```python
from build123d import *

# Parameters (mm, degrees)
SKETCH1_R           = 18.5
BOSS_EXTRUDE1_DEPTH = 26.5
SKETCH2_R           = 13.7
BOSS_EXTRUDE2_DEPTH = 38
SKETCH3_R           = 6
BOSS_EXTRUDE3_DEPTH = 6.8
SKETCH4_R           = 3
BOSS_EXTRUDE4_DEPTH = 30
SKETCH5_R           = 1.5
CUT_EXTRUDE1_DEPTH  = 6
CIRPATTERN1_COUNT   = 6
SKETCH6_R           = 13.75
BOSS_EXTRUDE5_DEPTH = 15
SKETCH7_R           = 1.5
CUT_EXTRUDE2_DEPTH  = 69.49372234


with BuildPart() as part:
    # Sketch1 → Boss-Extrude1 (new body)
    with BuildSketch(Plane.XY):
        Circle(SKETCH1_R)
    extrude(amount=BOSS_EXTRUDE1_DEPTH)

    # Sketch2 → Boss-Extrude2 (add)
    with BuildSketch(Plane(origin=(0, 0, 0), x_dir=(-1, 0, 0), z_dir=(0, 0, -1))):
        with Locations(Location((0, 0, 0), (0, 0, 180))):
            Circle(SKETCH2_R)
    extrude(amount=BOSS_EXTRUDE2_DEPTH)

    # Sketch3 → Boss-Extrude3 (add)
    with BuildSketch(Plane.XY.offset(26.5)):
        with Locations((0, 7)):
            Circle(SKETCH3_R)
    extrude(amount=BOSS_EXTRUDE3_DEPTH)

    # Sketch4 → Boss-Extrude4 (add)
    with BuildSketch(Plane.XY.offset(33.3)):
        with Locations((0, 7)):
            Circle(SKETCH4_R)
    extrude(amount=BOSS_EXTRUDE4_DEPTH)

    # Sketch5 → Cut-Extrude1 (cut)
    with BuildSketch(Plane.XY.offset(26.5)):
        with Locations((15.75, 0)):
            Circle(SKETCH5_R)
    cut_extrude1 = extrude(amount=-CUT_EXTRUDE1_DEPTH, mode=Mode.SUBTRACT)

    # CirPattern1: Cut-Extrude1 ×6 about axis
    cirpattern1_axis = Axis((0, 0, 0), (0, 0, 1))
    for i in range(1, CIRPATTERN1_COUNT):
        add(cut_extrude1.rotate(cirpattern1_axis, i * 360 / CIRPATTERN1_COUNT), mode=Mode.SUBTRACT)

    # Sketch6 → Boss-Extrude5 (add)
    with BuildSketch(Plane(origin=(0, 0, -38), x_dir=(-1, 0, 0), z_dir=(0, 0, -1))):
        Circle(SKETCH6_R)
    extrude(amount=BOSS_EXTRUDE5_DEPTH)

    # Sketch7 → Cut-Extrude2 (cut, through all)
    with BuildSketch(Plane(origin=(0, 0, 0), x_dir=(1, 0, 0), z_dir=(0, 1, 0))):
        with Locations(Location((0, -53.3, 0), (0, 0, 90))):
            Circle(SKETCH7_R)
    extrude(amount=CUT_EXTRUDE2_DEPTH, mode=Mode.SUBTRACT)


solid = part.part
```
The model under review builds one solid part; all positions refer to its coordinate system, in mm. A direction names the side the tool comes from. Round coordinates to 2 decimals unless told otherwise and drop trailing zeros. Write each loop counter-clockwise with the first axis right and the second up, starting at its lowest first coordinate (ties: lowest second). Pieces come first, ordered by that corner, then holes. Notation, with made-up numbers: (47.5, 34) - (74.5, 34) arc R3 ccw to (74.5, 39) - close; hole circle Ø1 at (26.5, -37). An arc over 180 degrees is marked (long way). Use one line per item in the form item = value.
Q1. For line 1 (Z direction, x = -6.5, y = 6.5); line 2 (Z direction, x = 4.5, y = 14); line 3 (X direction, y = 8.5, z = 53.3), list the stretches that pass through material, from the lowest coordinate up. Write a range as [from, to].
Answer key:
line_1 = [-53, 26.5]
line_2 = [0, 26.5]
line_3 = [-2.6, -1.5], [1.5, 2.6]
Q2. Consider section A-A (x = 0). State the section outline as (y, z) points, and give its area (3 significant figures).
Answer key:
outline = (-18.5, 0) - (-13.7, 0) - (-13.7, -38) - (-13.75, -38) - (-13.75, -53) - (13.75, -53) - (13.75, -38) - (13.7, -38) - (13.7, 0) - (18.5, 0) - (18.5, 26.5) - (13, 26.5) - (13, 33.3) - (10, 33.3) - (10, 51.8) - (4, 51.8) - (4, 33.3) - (1, 33.3) - (1, 26.5) - (-18.5, 26.5) - close; (4, 54.8) - (10, 54.8) - (10, 63.3) - (4, 63.3) - close
area = 2,680 mm2
Q3. Consider section B-B (y = 7). State the section outline as (x, z) points, and give its area (3 significant figures).
Answer key:
outline = (-17.12, 0) - (-11.78, 0) - (-11.78, -38) - (-11.83, -38) - (-11.83, -53) - (11.83, -53) - (11.83, -38) - (11.78, -38) - (11.78, 0) - (17.12, 0) - (17.12, 26.5) - (6, 26.5) - (6, 33.3) - (3, 33.3) - (3, 63.3) - (-3, 63.3) - (-3, 33.3) - (-6, 33.3) - (-6, 26.5) - (-17.12, 26.5) - close; hole circle Ø3 at (0, 53.3)
area = 2,410 mm2
Q4. Draft analysis for pull direction Z (two halves, no side actions). For faces 1 (the cylindrical face through (-1.265, 6.958, 52.494)), 2 (the flat face through (8, 14, 20.5)), state which applies: +Z half, -Z half, draft (parallel to the pull), parting line (faces both ways), or undercut.
Answer key:
face_1 = undercut
face_2 = +Z half
Q5. Consider section C-C (x = -10.5). State the section outline as (y, z) points.
Answer key:
outline = (-15.23, 0) - (-8.8, 0) - (-8.8, -38) - (-8.88, -38) - (-8.88, -53) - (8.88, -53) - (8.88, -38) - (8.8, -38) - (8.8, 0) - (15.23, 0) - (15.23, 26.5) - (-15.23, 26.5) - close
Q6. Tool access review of faces 3 (the cylindrical face through (-3, 7, 48)), 4 (the cylindrical face through (-4.01, -18.06, 13.06)): name each direction out of +Z, -Z, +X, -X, +Y, -Y from which nothing blocks a thin tool from reaching the whole face with its end or side.
Answer key:
face_3 = +Z
face_4 = +Z, -Z
Q7. Insertion check: pin 1 Ø2.5 at (x, y) = (-7.88, -13.64) entering from -Z; pin 2 Ø2.5 at (x, z) = (0, 53.3) entering from +Y; pin 3 Ø5 at (x, y) = (-15.75, 0) entering from +Z; pin 4 Ø10 at (x, z) = (8.5, -24) entering from +Y. Each pin has a flat end and moves straight along its axis. Give the tip position at first contact, or say it passes through.
Answer key:
pin_1 = 0
pin_2 = through
pin_3 = 26.5
pin_4 = 13.25
Q8. Consider section D-D (z = 53.3). State the section outline as (x, y) points, and give its area (3 significant figures).
Answer key:
outline = (-1.5, 4.4) - (-1.5, 9.6) arc R3 ccw to start; (1.5, 4.4) arc R3 ccw to (1.5, 9.6) - close
area = 11.1 mm2
